Design review of the part built by this model. Coordinates are the model's own, in mm. Face numbers are marked on the shaded views. A direction names the side the tool comes from. Give positions to 0.01 mm unless a question says otherwise; leave off trailing zeros. Order: outer loops, then holes, each group sorted by start corner. A loop starts at its lowest first (then second) coordinate and runs counter-clockwise, first axis right, second up. Notation, with made-up numbers: (44.5, 45.5) -> (54.5, 45.5) arc R13 ccw to (54.5, 58.5) -> close; hole circle Ø10 at (46.5, 59). An arc over 180 degrees is marked (long way). Answer in a Markdown table with one row per item. Add a question column.
Autodesk Inventor part; units mm, degrees
ref_plane "YZ Plane" through (0, 0, 0) normal (1, 0, 0) x (0, 1, 0)
ref_plane "XZ Plane" through (0, 0, 0) normal (0, 1, 0) x (-1, 0, 0)
ref_plane "XY Plane" through (0, 0, 0) normal (0, 0, 1) x (1, 0, 0)
sketch "Sketch1" plane through (0, 0, 0) normal (0, 1, 0) x (-1, 0, 0)
  circle A0 centre (0, 0) radius 3.5
  dimension "d0" = 7
extrude "Extrusion1" add sketch "Sketch1" along normal blind 5
sketch "Sketch2" plane through (0, 5, 0) normal (0, 1, 0) x (1, 0, 0)
  line L0 (-1.8, -1.8) -> (1.8, -1.8)
  line L1 (1.8, -1.8) -> (1.8, 1.8)
  line L2 (1.8, 1.8) -> (-1.8, 1.8)
  line L3 (-1.8, 1.8) -> (-1.8, -1.8)
  point P0 (0, 0)
  dimension "d3" = 3.6
  dimension "d4" = 3.6
  dimension "d5" = 1.8
  dimension "d6" = 1.8
extrude "Extrusion2" cut sketch "Sketch2" against normal blind 2
sketch "Sketch3" plane through (0, 3, 0) normal (0, 1, 0) x (1, 0, 0)
  circle A0 centre (0, 0) radius 1.5
  dimension "d9" = 3
extrude "Extrusion3" cut sketch "Sketch3" against normal through all
fillet "Fillet1" radius 0.9 1 edges at (-1.5, 3, 0)
properties part number "LED8SUPPORT"
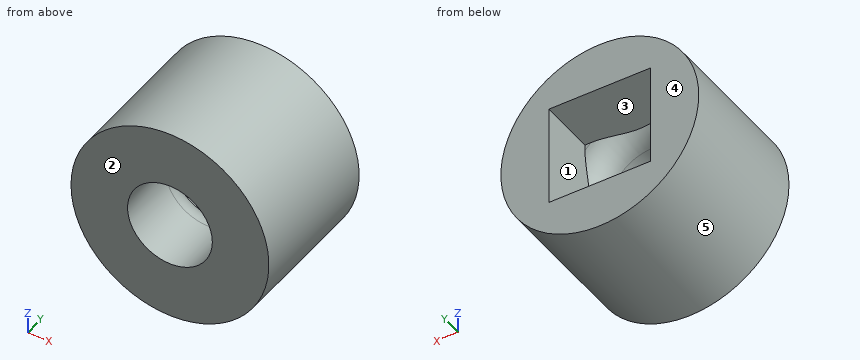
1) Machinability: for the marked faces 1 and 2, which of the approach directions +Z, -Z, +X, -X, +Y, -Y give a long, thin tool a straight path to every point of the face, cutting with its end or side? Answer none if there is none.
2) Mouldability with a two-part tool opening along X and no side actions: class the marked faces 3, 4 and 5 as +X half, -X half, draft (parallel to the pull), parting line (faces both ways), or undercut.
3) Add section B-B, the plane z = 0. Write out the cut boundary in (x, y), and give its area (3 significant figures).
4) Add section C-C, the plane y = 3.1. Write out the cut boundary in (x, z).
5) Add section D-D, the plane y = 1.8. Write out the cut boundary in (x, z), and give its area (3 significant figures).
6) Add section A-A, the plane x = 0. Write out the cut boundary in (y, z).
7) Clearance check with flat-ended pins moving along their axes: P1, Ø1.8, axis at x = 0.5, y = 4, coming from the +Z side; P2, Ø0.7, axis at y = 4, z = -0.5, coming from the +X side; P3, Ø1.5, axis at y = 2.5, z = -1, coming from the -X side. State where each tip first meets the part, or that it passes through.
8) For L1, parallel to Z at x = 0, y = 0.7; L2, parallel to X at y = 2.4, z = -0.25; L3, parallel to X at y = 0.65, z = 0.5, list the stretches that pass through material, from the lowest coordinate up.
Verdict:
| question | item | result |
|---|---|---|
| 1 | face 1 | +Y |
| 1 | face 2 | +Z, -Z, +X, -X, -Y |
| 2 | face 3 | undercut |
| 2 | face 4 | draft |
| 2 | face 5 | parting line |
| 3 | outline | (-3.5, 0) -> (-1.5, 0) -> (-1.5, 2.1) arc R0.9 ccw to (-1.8, 2.77) -> (-1.8, 5) -> (-3.5, 5) -> close; (1.5, 0) -> (3.5, 0) -> (3.5, 5) -> (1.8, 5) -> (1.8, 2.77) arc R0.9 ccw to (1.5, 2.1) -> close |
| 3 | area | 18.5 mm2 |
| 4 | outline | circle Ø7 at (0, 0); hole (-1.8, -1.8) -> (1.8, -1.8) -> (1.8, 1.8) -> (-1.8, 1.8) -> close |
| 5 | outline | circle Ø7 at (0, 0); hole circle Ø3 at (0, 0) |
| 5 | area | 31.4 mm2 |
| 6 | outline | (0, -3.5) -> (5, -3.5) -> (5, -1.8) -> (2.77, -1.8) arc R0.9 ccw to (2.1, -1.5) -> (0, -1.5) -> close; (0, 1.5) -> (2.1, 1.5) arc R0.9 ccw to (2.77, 1.8) -> (5, 1.8) -> (5, 3.5) -> (0, 3.5) -> close |
| 7 | P1 | stops at z = 3.5 |
| 7 | P2 | stops at x = 3.5 |
| 7 | P3 | stops at x = -3.49 |
| 8 | L1 | z = -3.5 to -1.5, 1.5 to 3.5 |
| 8 | L2 | x = -3.49 to -1.53, 1.53 to 3.49 |
| 8 | L3 | x = -3.46 to -1.41, 1.41 to 3.46 |
